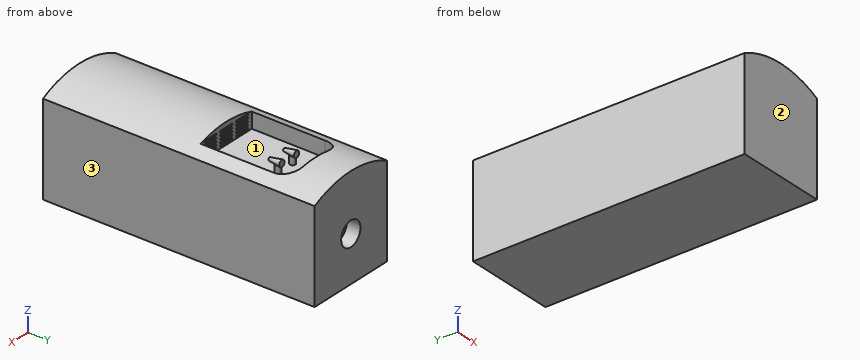
```python
from build123d import *

# Parameters (mm, degrees)
BOSS_EXTRUDE1_DEPTH = 127
CUT_EXTRUDE1_DEPTH  = 88.9
CUT_EXTRUDE2_DEPTH  = 1.27
CUT_EXTRUDE3_DEPTH  = 6.35
SKETCH6_R           = 1.27
BOSS_EXTRUDE2_DEPTH = 3.81
SCALE1_SCALE        = 10
SCALE2_SCALE        = 0.8


with BuildPart() as part:
    # Sketch1 → Boss-Extrude1 (new body)
    with BuildSketch(Plane(origin=(0, 0, 0), x_dir=(1, 0, 0), z_dir=(0, 1, 0))):
        with BuildLine():
            Line((0, 0), (42.739614803, 0))
            Line((42.739614803, 0), (42.739614803, -42.739614803))
            ThreePointArc((42.739614803, -42.739614803), (21.369807402, -47.941054373), (0, -42.739614803))
            Line((0, -42.739614803), (0, 0))
        make_face()
    extrude(amount=BOSS_EXTRUDE1_DEPTH)

    # Sketch2 → Cut-Extrude1 (cut)
    with BuildSketch(Plane.XY.offset(127)):
        with BuildLine():
            Line((13.881687598, 110.608783011), (28.857927206, 110.608783011))
            ThreePointArc((28.857927206, 110.608783011), (34.246080878, 108.376936683), (36.477927206, 102.988783011))
            Line((36.477927206, 102.988783011), (36.477927206, 68.734309223))
            Line((36.477927206, 68.734309223), (6.261687598, 68.734309223))
            Line((6.261687598, 68.734309223), (6.261687598, 102.988783011))
            ThreePointArc((6.261687598, 102.988783011), (8.493533925, 108.376936683), (13.881687598, 110.608783011))
        make_face()
    extrude(amount=-CUT_EXTRUDE1_DEPTH, mode=Mode.SUBTRACT)

    # Sketch4 → Cut-Extrude2 (cut)
    with BuildSketch(Plane(origin=(0, 68.734309223, 0), x_dir=(1, 0, 0), z_dir=(0, 1, 0))):
        with BuildLine():
            Line((18.101107041, -45.607119247), (24.638507762, -45.607119247))
            ThreePointArc((24.638507762, -45.607119247), (25.019507762, -45.226119247), (24.638507762, -44.845119247))
            Line((24.638507762, -44.845119247), (18.101107041, -44.845119247))
            ThreePointArc((18.101107041, -44.845119247), (17.720107041, -45.226119247), (18.101107041, -45.607119247))
        make_face()
        with BuildLine():
            Line((8.722196959, -45.607119247), (15.25959768, -45.607119247))
            ThreePointArc((15.25959768, -45.607119247), (15.64059768, -45.226119247), (15.25959768, -44.845119247))
            Line((15.25959768, -44.845119247), (8.722196959, -44.845119247))
            ThreePointArc((8.722196959, -44.845119247), (8.341196959, -45.226119247), (8.722196959, -45.607119247))
        make_face()
        with BuildLine():
            Line((8.722196959, -42.559119247), (15.25959768, -42.559119247))
            ThreePointArc((15.25959768, -42.559119247), (15.64059768, -42.178119247), (15.25959768, -41.797119247))
            Line((15.25959768, -41.797119247), (8.722196959, -41.797119247))
            ThreePointArc((8.722196959, -41.797119247), (8.341196959, -42.178119247), (8.722196959, -42.559119247))
        make_face()
        with BuildLine():
            Line((8.722196959, -44.083119247), (15.25959768, -44.083119247))
            ThreePointArc((15.25959768, -44.083119247), (15.64059768, -43.702119247), (15.25959768, -43.321119247))
            Line((15.25959768, -43.321119247), (8.722196959, -43.321119247))
            ThreePointArc((8.722196959, -43.321119247), (8.341196959, -43.702119247), (8.722196959, -44.083119247))
        make_face()
        with BuildLine():
            Line((18.101107041, -44.083119247), (24.638507762, -44.083119247))
            ThreePointArc((24.638507762, -44.083119247), (25.019507762, -43.702119247), (24.638507762, -43.321119247))
            Line((24.638507762, -43.321119247), (18.101107041, -43.321119247))
            ThreePointArc((18.101107041, -43.321119247), (17.720107041, -43.702119247), (18.101107041, -44.083119247))
        make_face()
        with BuildLine():
            Line((18.101107041, -42.559119247), (24.638507762, -42.559119247))
            ThreePointArc((24.638507762, -42.559119247), (25.019507762, -42.178119247), (24.638507762, -41.797119247))
            Line((24.638507762, -41.797119247), (18.101107041, -41.797119247))
            ThreePointArc((18.101107041, -41.797119247), (17.720107041, -42.178119247), (18.101107041, -42.559119247))
        make_face()
        with BuildLine():
            Line((18.101107041, -41.035119247), (24.638507762, -41.035119247))
            ThreePointArc((24.638507762, -41.035119247), (25.019507762, -40.654119247), (24.638507762, -40.273119247))
            Line((24.638507762, -40.273119247), (18.101107041, -40.273119247))
            ThreePointArc((18.101107041, -40.273119247), (17.720107041, -40.654119247), (18.101107041, -41.035119247))
        make_face()
        with BuildLine():
            Line((18.101107041, -39.511119247), (24.638507762, -39.511119247))
            ThreePointArc((24.638507762, -39.511119247), (25.019507762, -39.130119247), (24.638507762, -38.749119247))
            Line((24.638507762, -38.749119247), (18.101107041, -38.749119247))
            ThreePointArc((18.101107041, -38.749119247), (17.720107041, -39.130119247), (18.101107041, -39.511119247))
        make_face()
        with BuildLine():
            Line((8.722196959, -41.035119247), (15.25959768, -41.035119247))
            ThreePointArc((15.25959768, -41.035119247), (15.64059768, -40.654119247), (15.25959768, -40.273119247))
            Line((15.25959768, -40.273119247), (8.722196959, -40.273119247))
            ThreePointArc((8.722196959, -40.273119247), (8.341196959, -40.654119247), (8.722196959, -41.035119247))
        make_face()
        with BuildLine():
            Line((8.722196959, -39.511119247), (15.25959768, -39.511119247))
            ThreePointArc((15.25959768, -39.511119247), (15.64059768, -39.130119247), (15.25959768, -38.749119247))
            Line((15.25959768, -38.749119247), (8.722196959, -38.749119247))
            ThreePointArc((8.722196959, -38.749119247), (8.341196959, -39.130119247), (8.722196959, -39.511119247))
        make_face()
        with BuildLine():
            Line((27.480017123, -44.083119247), (34.017417844, -44.083119247))
            ThreePointArc((34.017417844, -44.083119247), (34.398417844, -43.702119247), (34.017417844, -43.321119247))
            Line((34.017417844, -43.321119247), (27.480017123, -43.321119247))
            ThreePointArc((27.480017123, -43.321119247), (27.099017123, -43.702119247), (27.480017123, -44.083119247))
        make_face()
        with BuildLine():
            Line((27.480017123, -42.559119247), (34.017417844, -42.559119247))
            ThreePointArc((34.017417844, -42.559119247), (34.398417844, -42.178119247), (34.017417844, -41.797119247))
            Line((34.017417844, -41.797119247), (27.480017123, -41.797119247))
            ThreePointArc((27.480017123, -41.797119247), (27.099017123, -42.178119247), (27.480017123, -42.559119247))
        make_face()
        with BuildLine():
            Line((27.480017123, -41.035119247), (34.017417844, -41.035119247))
            ThreePointArc((34.017417844, -41.035119247), (34.398417844, -40.654119247), (34.017417844, -40.273119247))
            Line((34.017417844, -40.273119247), (27.480017123, -40.273119247))
            ThreePointArc((27.480017123, -40.273119247), (27.099017123, -40.654119247), (27.480017123, -41.035119247))
        make_face()
        with BuildLine():
            Line((27.480017123, -39.511119247), (34.017417844, -39.511119247))
            ThreePointArc((34.017417844, -39.511119247), (34.398417844, -39.130119247), (34.017417844, -38.749119247))
            Line((34.017417844, -38.749119247), (27.480017123, -38.749119247))
            ThreePointArc((27.480017123, -38.749119247), (27.099017123, -39.130119247), (27.480017123, -39.511119247))
        make_face()
        with BuildLine():
            ThreePointArc((27.480017123, -44.845119247), (27.099017123, -45.226119247), (27.480017123, -45.607119247))
            Line((27.480017123, -45.607119247), (34.017417844, -45.607119247))
            ThreePointArc((34.017417844, -45.607119247), (34.398417844, -45.226119247), (34.017417844, -44.845119247))
            Line((34.017417844, -44.845119247), (27.480017123, -44.845119247))
        make_face()
    extrude(amount=-CUT_EXTRUDE2_DEPTH, mode=Mode.SUBTRACT)

    # Sketch5 → Cut-Extrude3 (cut)
    with BuildSketch(Plane(origin=(0, 127, 0), x_dir=(1, 0, 0), z_dir=(0, 1, 0))):
        with BuildLine():
            ThreePointArc((27.058825704, -21.369807402), (21.369807402, -15.680789099), (15.680789099, -21.369807402))
            Line((15.680789099, -21.369807402), (27.058825704, -21.369807402))
        make_face()
        with BuildLine():
            Line((27.058825704, -21.369807402), (15.680789099, -21.369807402))
            ThreePointArc((15.680789099, -21.369807402), (21.369807402, -27.058825704), (27.058825704, -21.369807402))
        make_face()
    extrude(amount=-CUT_EXTRUDE3_DEPTH, mode=Mode.SUBTRACT)

    # Sketch6 → Boss-Extrude2 (add)
    with BuildSketch(Plane.XY.offset(38.1)):
        with Locations(Location((17.026937254, 96.316061715, 0), (0, 0, 180))):
            Circle(SKETCH6_R)
        with Locations(Location((25.712677549, 96.316061715, 0), (0, 0, 180))):
            Circle(SKETCH6_R)
    extrude(amount=BOSS_EXTRUDE2_DEPTH)

    # Sketch8 → Revolve1 (revolve)
    with BuildSketch(Plane.YZ.offset(17.026937254), mode=Mode.PRIVATE) as revolve1_sk:
        Polygon((92.462776609, 42.625909045), (92.462776609, 43.341818089), (98.173073883, 44.293534302), (98.173073883, 42.739614803), align=None)
    revolve1 = revolve(revolve1_sk.sketch.rotate(Axis((17.026937254, 92.462776609, 42.625909045), (0, 0.9998018069764348, 0.01990845967561906)), 180), axis=Axis((17.026937254, 92.462776609, 42.625909045), (0, 0.9998018069764348, 0.01990845967561906)))

    # Mirror1: Revolve1 across plane
    add(revolve1.mirror(Plane.ZY.offset(-21.369807402)))


with BuildPart() as part_1:
    # Scale1: scaled about (21.369807188, 62.136257344, 22.239140039)
    add(part.part.scale(SCALE1_SCALE).moved(Location((-192.328264692, -559.226316096, -200.152260351))))


with BuildPart() as part_2:
    # Scale2: scaled about (21.369807187, 62.136257344, 22.239140034)
    add(part_1.part.scale(SCALE2_SCALE).moved(Location((4.273961437, 12.427251469, 4.447828007))))


solid = part_2.part
```
Input: part model. Units: mm. Frame: model coordinates. Face numbers are marked on the shaded views. Coordinates: 2 decimals unless noted, no trailing zeros. Write each loop counter-clockwise with the first axis right and the second up, starting at its lowest first coordinate (ties: lowest second). Pieces come first, ordered by that corner, then holes. Notation, with made-up numbers: (11.25, -9) - (43.25, -9) arc R28 cw to (43.25, 15) - close; hole circle Ø3 at (75, 79.5). An arc over 180 degrees is marked (long way). Put each result on its own line as item: value. Start each with the question number.
1) Cut plane B-B (x = 91.5). Return the cut outline in (y, z), plus the area to 3 significant figures.
2) Contact query for flat-ended pins moving along their axis: pin 1 (1.5 mm diameter, centred on x = 144, y = 233, fed in from +Z); pin 2 (8 mm diameter, centred on x = -49.5, y = 109.5, fed in from +Z); pin 3 (11 mm diameter, centred on x = 99.5, y = 112, fed in from +Z). Output: stop coordinate, or through.
3) Mould query, pull axis X, two halves, no side actions, for the marked faces 1, 2 and 3. Classes: pulls with the +X half, pulls with the -X half, needs draft (parallel to the pull), parting line crosses it, or undercut.
4) Cut plane D-D (y = 419). Return the cut outline in (x, z), plus the area to 3 significant figures.
5) Ray query, L1, parallel to Z at x = 134, y = 164.5; L2, parallel to Z at x = 171.5, y = -269.5. Return the intervals inside material, ascending.
6) Cut plane A-A (y = 233). Return the cut outline in (x, z).
7) Cut plane C-C (x = -66). Return the cut outline in (y, z), plus the area to 3 significant figures.
Resolved:
1. outline: (-434.95, -155.67) - (581.05, -155.67) - (581.05, 221.18) - (449.05, 221.18) - (449.05, 149.13) - (114.92, 149.13) - (114.92, 154.32) - (104.76, 154.32) - (104.76, 160.41) - (114.92, 160.41) - (114.92, 166.51) - (104.76, 166.51) - (104.76, 172.61) - (114.92, 172.61) - (114.92, 178.7) - (104.76, 178.7) - (104.76, 184.8) - (114.92, 184.8) - (114.92, 190.89) - (104.76, 190.89) - (104.76, 196.99) - (114.92, 196.99) - (114.92, 203.09) - (104.76, 203.09) - (104.76, 209.18) - (114.92, 209.18) - (114.92, 221.18) - (-434.95, 221.18) - close
1. area: 359,000 mm2
2. pin 1: stops at z = 207.32
2. pin 2: stops at z = 221.79
2. pin 3: stops at z = 220.7
3. face 1: undercut
3. face 2: needs draft
3. face 3: pulls with the +X half
4. outline: (-149.59, -155.67) - (192.33, -155.67) - (192.33, 186.24) arc R371.99 ccw to (134.32, 210.29) - (134.32, 149.13) - (-91.58, 149.13) - (-91.58, 210.29) arc R371.99 ccw to (-149.59, 186.24) - close
4. area: 110,000 mm2
5. L1: z = -155.67 to 149.13
5. L2: z = -155.67 to 196.21
6. outline: (-149.59, -155.67) - (192.33, -155.67) - (192.33, 186.24) arc R371.99 ccw to (142.23, 207.67) - (142.23, 149.13) - (-99.5, 149.13) - (-99.5, 207.67) arc R371.99 ccw to (-149.59, 186.24) - close
7. outline: (-434.95, -155.67) - (581.05, -155.67) - (581.05, 217.45) - (443.38, 217.45) - (443.38, 149.13) - (114.92, 149.13) - (114.92, 154.32) - (104.76, 154.32) - (104.76, 160.41) - (114.92, 160.41) - (114.92, 166.51) - (104.76, 166.51) - (104.76, 172.61) - (114.92, 172.61) - (114.92, 178.7) - (104.76, 178.7) - (104.76, 184.8) - (114.92, 184.8) - (114.92, 190.89) - (104.76, 190.89) - (104.76, 196.99) - (114.92, 196.99) - (114.92, 203.09) - (104.76, 203.09) - (104.76, 209.18) - (114.92, 209.18) - (114.92, 217.45) - (-434.95, 217.45) - close
7. area: 356,000 mm2
